Source: CAD feature listing. Evaluate the final solid. Frame: model axes, mm. Face numbers are marked on the shaded views. A direction names the side the tool comes from. Coordinates: 2 decimals unless noted, no trailing zeros. Loops run counter-clockwise (first coordinate to the right, second up) from the corner with the lowest first, then second, coordinate; pieces in that order, holes last. Notation, with made-up numbers: (-2, 87.5) - (53, 87.5) arc R11 ccw to (53, 100.5) - close; hole circle Ø11 at (17.5, -40). An arc over 180 degrees is marked (long way). Use CSV: the item, a comma, the result in double quotes. Start each with the question number.
```python
from build123d import *

# Parameters (mm, degrees)
SALIENTE_EXTRUIR1_DEPTH = 338.5
VACIADO1_T              = -20
SALIENTE_EXTRUIR2_DEPTH = 10
MATRIZL1_COUNT          = 2
MATRIZL1_PITCH          = 170
MATRIZL2_COUNT          = 2
MATRIZL2_PITCH          = 170


with BuildPart() as part:
    # Croquis1 → Saliente-Extruir1 (new, symmetric)
    with BuildSketch(Plane.XY):
        Polygon((0, 0), (0, 50), (1160.4, 151.521845155), (1160.4, 0), align=None)
    extrude(amount=SALIENTE_EXTRUIR1_DEPTH, both=True)

    # Vaciado1
    vaciado1_openings = [part.faces().sort_by_distance(p)[0] for p in [
        (580.2, 0, 0),
    ]]
    offset(amount=VACIADO1_T, openings=vaciado1_openings, kind=Kind.INTERSECTION)

    # Croquis2 → Saliente-Extruir2 (add, symmetric)
    with BuildSketch(Plane.XY):
        Polygon((20, 31.67337652), (20, 0), (1140.4, 0), (1140.4, 129.695675134), align=None)
    saliente_extruir2 = extrude(amount=SALIENTE_EXTRUIR2_DEPTH, both=True)

    # MatrizL1: Saliente-Extruir2 ×2
    with Locations(*[(0, 0, i * MATRIZL1_PITCH) for i in range(1, MATRIZL1_COUNT)]):
        add(saliente_extruir2)

    # MatrizL2: Saliente-Extruir2 ×2
    with Locations(*[(0, 0, -i * MATRIZL2_PITCH) for i in range(1, MATRIZL2_COUNT)]):
        add(saliente_extruir2)


solid = part.part
```
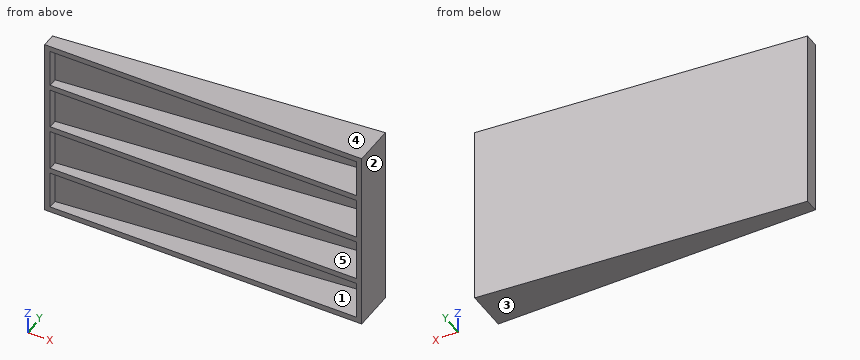
(1) Reachability of the marked faces 4 and 5 from +Z, -Z, +X, -X, +Y, -Y: full face, straight path, thin tool, end or side. Return the list, or none.
(2) Section A-A on y = 14. Output: boundary loops of the cut face in (x, z), plus the area to 3 significant figures.
(3) Section D-D on x = 251.5. Output: boundary loops of the cut face in (y, z).
(4) Section B-B on z = 245. Output: boundary loops of the cut face in (x, y), plus the area to 3 significant figures.
(5) Pin query (flat end, axial travel): pin 1 Ø5 at (x, z) = (894.5, 80.5) entering from +Y; pin 2 Ø1.5 at (x, z) = (979, 204) entering from +Y; pin 3 Ø10 at (x, z) = (672, -190.5) entering from +Y. Return the tip coordinate at first contact, or that it passes through.
(6) Ray query, line 1 (Z direction, x = 921, y = 53.5); line 2 (Y direction, x = 910, z = -175); line 3 (Y direction, x = 1016.5, z = 93). Return the intervals inside material, ascending. Write a range as [from, to].
(7) Draft query along Z for the marked faces 1, 2 and 3. Return one class per face: released by +Z, released by -Z, zero draft, split by the parting line, or undercut.
(8) Section C-C on x = 106. Output: boundary loops of the cut face in (y, z), plus the area to 3 significant figures.
Solution:
1,face 4,"+Z, +X, -X, +Y, -Y"
1,face 5,"-Y"
2,outline,"(0, -338.5) - (1160.4, -338.5) - (1160.4, 338.5) - (0, 338.5) - close; hole (20, -318.5) - (1140.4, -318.5) - (1140.4, -180) - (20, -180) - close; hole (20, -160) - (1140.4, -160) - (1140.4, -10) - (20, -10) - close; hole (20, 10) - (1140.4, 10) - (1140.4, 160) - (20, 160) - close; hole (20, 180) - (1140.4, 180) - (1140.4, 318.5) - (20, 318.5) - close"
2,area,"139,000 mm²"
3,outline,"(0, -338.5) - (72, -338.5) - (72, 338.5) - (0, 338.5) - (0, 318.5) - (51.93, 318.5) - (51.93, 180) - (0, 180) - (0, 160) - (51.93, 160) - (51.93, 10) - (0, 10) - (0, -10) - (51.93, -10) - (51.93, -160) - (0, -160) - (0, -180) - (51.93, -180) - (51.93, -318.5) - (0, -318.5) - close"
4,outline,"(0, 0) - (20, 0) - (20, 31.67) - (1140.4, 129.7) - (1140.4, 0) - (1160.4, 0) - (1160.4, 151.52) - (0, 50) - close"
4,area,"26,500 mm²"
5,pin 1,"stops at y = 128.48"
5,pin 2,"stops at y = 135.72"
5,pin 3,"stops at y = 109.23"
6,line 1,"z = [-338.5, -318.5], [-180, -160], [-10, 10], [160, 180], [318.5, 338.5]"
6,line 2,"y = [0, 129.61]"
6,line 3,"y = [118.86, 138.93]"
7,face 1,"undercut"
7,face 2,"zero draft"
7,face 3,"released by -Z"
8,outline,"(0, -338.5) - (59.27, -338.5) - (59.27, 338.5) - (0, 338.5) - (0, 318.5) - (39.2, 318.5) - (39.2, 180) - (0, 180) - (0, 160) - (39.2, 160) - (39.2, 10) - (0, 10) - (0, -10) - (39.2, -10) - (39.2, -160) - (0, -160) - (0, -180) - (39.2, -180) - (39.2, -318.5) - (0, -318.5) - close"
8,area,"17,500 mm²"
